Can you work these out from the drawing? Everything is in mm from the part's minimum corner. A direction names the side the tool comes from. Round coordinates to 2 decimals unless told otherwise and drop trailing zeros. Loops run counter-clockwise (first coordinate to the right, second up) from the corner with the lowest first, then second, coordinate; pieces in that order, holes last. Notation, with made-up numbers: M -1,-6.5 L 53,-6.5 A24 ccw 53,15.5 Z; hole C 21.25,82 d9. An arc over 180 degrees is marked long. Use a Markdown table: item, result.
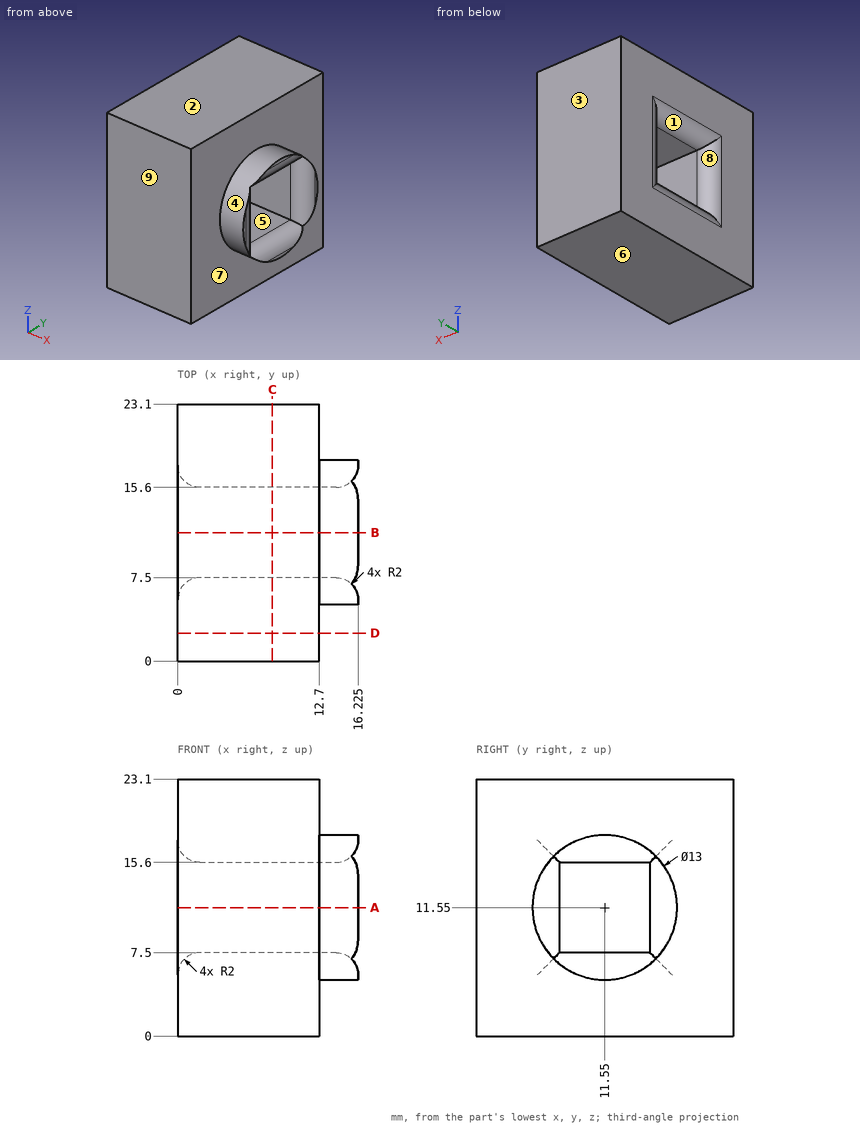
Q1. Imagine slicing it at D-D, the plane y = 2.5. Please give me the cut outline in (x, z).
Return value:
| item | result |
|---|---|
| outline | M 0,0 L 12.7,0 L 12.7,23.1 L 0,23.1 Z |
Q2. I need wall thicknesses on line 1 (Y direction, x = 2.75, z = 8); line 2 (X direction, y = 1, z = 14.25). Which ranges of each line are inside material? Lowest first, please. Write a range as from..to.
Return value:
| item | result |
|---|---|
| line 1 | y = 0..7.5, 15.6..23.1 |
| line 2 | x = 0..12.7 |
Q3. Imagine slicing it at C-C, the plane x = 8.5. Please give me the cut outline in (y, z).
Return value:
| item | result |
|---|---|
| outline | M 0,0 L 23.1,0 L 23.1,23.1 L 0,23.1 Z; hole M 7.5,7.5 L 15.6,7.5 L 15.6,15.6 L 7.5,15.6 Z |
Q4. Will these pins go through, and if not, where does the flat tip stop? P1, Ø5, axis at y = 20, z = 17, coming from the +X side; P2, Ø4, axis at x = 5, y = 11.5, coming from the -Z side; P3, Ø8, axis at y = 11, z = 13.5, coming from the -X side; P4, Ø3, axis at x = 14.5, y = 14, coming from the +Z side.
Return value:
| item | result |
|---|---|
| P1 | stops at x = 12.7 |
| P2 | stops at z = 0 |
| P3 | stops at x = 0 |
| P4 | stops at z = 17.98 |
Q5. For the marked faces 5, 6, 7, 8 and 9, which set-ups out of +Z, -Z, +X, -X, +Y, -Y let a thin tool reach every point of the face, with its end or its side?
Return value:
| item | result |
|---|---|
| face 5 | +X, -X |
| face 6 | -Z, +X, -X, +Y, -Y |
| face 7 | +X |
| face 8 | -X |
| face 9 | +Z, -Z, +X, -X, -Y |
Q6. Imagine slicing it at A-A, the plane z = 11.55. Please give me the cut outline in (x, y) (3 decimals), then the cut area to 3 significant figures.
Return value:
| item | result |
|---|---|
| outline | M 0,0 L 12.7,0 L 12.7,5.05 L 16.225,5.05 L 16.225,5.5 A2 ccw 14.225,7.5 L 2,7.5 A2 ccw 0,5.5 Z; M 0,17.6 A2 ccw 2,15.6 L 14.225,15.6 A2 ccw 16.225,17.6 L 16.225,18.05 L 12.7,18.05 L 12.7,23.1 L 0,23.1 Z |
| area | 204 mm^2 |
Q7. We'd pull the mould along Y, two halves only. Please class the marked faces 1, 2, 3 and 4: pulls with the +Y half, pulls with the -Y half, needs draft (parallel to the pull), parting line crosses it, or undercut.
Return value:
| item | result |
|---|---|
| face 1 | undercut |
| face 2 | needs draft |
| face 3 | pulls with the +Y half |
| face 4 | parting line crosses it |
